Can you work these out from the model? Positions are in its coordinate system, mm. Face numbers are marked on the shaded views. A direction names the side the tool comes from. Coordinates: 2 decimals unless noted, no trailing zeros. Order: outer loops, then holes, each group sorted by start corner. A loop starts at its lowest first (then second) coordinate and runs counter-clockwise, first axis right, second up. Notation, with made-up numbers: (82.25, 80.5) - (102.25, 80.5) arc R19 ccw to (102.25, 113.5) - close; hole circle Ø4 at (16.5, 70.5). An arc over 180 degrees is marked (long way). Use a Markdown table: item, result. Add a question column.
(1) I want a section at B-B (y = 0). List the corners of the cut face in (x, z) for me (3 decimals), and give its area (3 significant figures).
(2) If I drill on L1, parallel to Y at x = 0, z = 15.5; L2, parallel to Z at x = 0, y = 11.5; L3, parallel to Z at x = -14.5, y = -59.5, over which ranges is the centre line in solid material (lowest first)? Write a range as [from, to].
(3) On a 3-axis mill with a long thin cutter (end or side, diameter ignored), from which of +Z, -Z, +X, -X, +Y, -Y can I reach the whole of each face in a straight line? I mean the marked faces 1, 2 and 3. Say none if no direction works.
(4) I want a section at C-C (z = 18). List the corners of the cut face in (x, y) for me.
(5) For pin 1 Ø8 at (y, z) = (32.5, 3) entering from +X; pin 2 Ø16 at (x, y) = (-2.5, -0.5) entering from +Z; pin 3 Ø8 at (y, z) = (-7.5, -5) entering from -X, each with a flat end and sliding along its axis, tell me the tip position at first contact or that it passes through.
(6) I want a section at D-D (z = -14). List the corners of the cut face in (x, y) for me.
Autodesk Inventor part; units mm, degrees
ref_plane "YZ Plane" through (0, 0, 0) normal (1, 0, 0) x (0, 1, 0)
ref_plane "XZ Plane" through (0, 0, 0) normal (0, 1, 0) x (-1, 0, 0)
ref_plane "XY Plane" through (0, 0, 0) normal (0, 0, 1) x (1, 0, 0)
sketch "草图1" plane through (0, 0, 0) normal (0, 0, 1) x (1, 0, 0)
  circle A0 centre (0, 0) radius 65
  dimension "d0" = 130
extrude "拉伸1" add sketch "草图1" along normal blind 12
sketch "草图2" plane through (0, 0, 12) normal (0, 0, 1) x (1, 0, 0)
  circle A0 centre (0, 0) radius 50
  circle A1 centre (0, 50) radius 7.5
  line L0 (0, 0) -> (0, 11.3897)
  dimension "d3" = 100
  dimension "d4" = 15
  dimension "d5" = 11.3897
extrude "拉伸2" add sketch "草图2" along normal blind 15 contours A1 A0 | A0 A1 picked at (0, 47.4583) picked at (0.2152, 52.449)
sketch "草图3" plane through (0, 50, 27) normal (0, 0, 1) x (1, 0, 0)
  circle A0 centre (0, 0) radius 2.5
  circle A1 centre (0, 0) radius 7.5
  point P0 (0, -50)
  dimension "d8" = 5
extrude "拉伸3" cut sketch "草图3" against normal through all contours A0
thread "螺纹1"
sketch "草图4" plane through (0, 0, 0) normal (0, 0, -1) x (-1, 0, 0)
  circle A0 centre (0, 0) radius 10
  dimension "d13" = 20
extrude "拉伸4" add sketch "草图4" along normal blind 59.7
sketch "草图5" plane through (0, 0, 0) normal (0, 0, -1) x (-1, 0, 0)
  circle A0 centre (0, 0) radius 13
  dimension "d16" = 26
extrude "拉伸5" add sketch "草图5" along normal blind 3
chamfer "倒角1" distance 2 angle 45 2 edges at (-65, 0, 0) (-65, 0, 12)
chamfer "倒角2" distance 0.5 angle 45 1 edges at (10, 0, -59.7)
sketch "草图6" plane through (0, 0, 0) normal (0, 1, 0) x (-1, 0, 0)
  line L0 (-9.175, -54.5) -> (-18.451, -54.5)
  line L1 (-18.451, -54.5) -> (-18.451, -55.7)
  line L2 (-18.451, -55.7) -> (-9.175, -55.7)
  line L3 (-9.175, -55.7) -> (-9.175, -54.5)
  line L4 (9.5, -59.7) -> (-9.5, -59.7)
  line L5 (0, -59.7) -> (0, -69.9932)
  point P0 (0, 0)
  dimension "d25" = 10.2932
  dimension "d26" = 4
  dimension "d27" = 1.2
  dimension "d28" = 9.175
  dimension "d29" = 9.276
revolve "旋转1" cut sketch "草图6" angle 360 about axis through (0, 0, -59.7) along (0, 0, -1)
properties part number "刀轴带动盘"
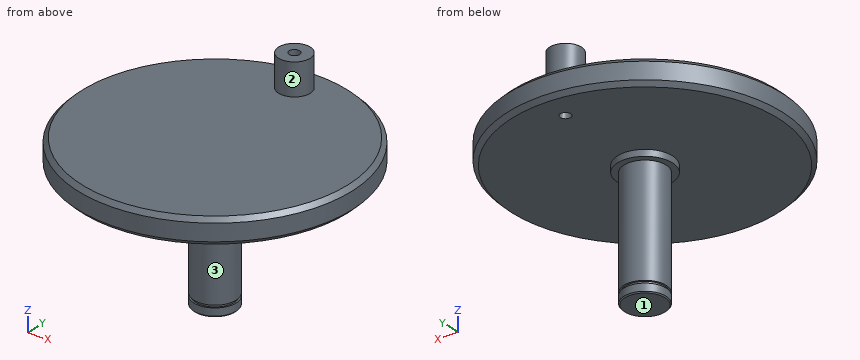
Answers follow:
| question | item | result |
|---|---|---|
| 1 | outline | (-65, 2) - (-63, 0) - (-13, 0) - (-13, -3) - (-10, -3) - (-10, -54.5) - (-9.175, -54.5) - (-9.175, -55.7) - (-10, -55.7) - (-10, -59.2) - (-9.5, -59.7) - (9.5, -59.7) - (10, -59.2) - (10, -55.7) - (9.175, -55.7) - (9.175, -54.5) - (10, -54.5) - (10, -3) - (13, -3) - (13, 0) - (63, 0) - (65, 2) - (65, 10) - (63, 12) - (-63, 12) - (-65, 10) - close |
| 1 | area | 2,760 mm² |
| 2 | L1 | y = [42.5, 47.5], [52.5, 57.5] |
| 2 | L2 | z = [-3, 12] |
| 2 | L3 | z = [0, 12] |
| 3 | face 1 | -Z, +X, -X, +Y, -Y |
| 3 | face 2 | +Z |
| 3 | face 3 | -Z |
| 4 | outline | circle Ø15 at (0, 50); hole circle Ø5 at (0, 50) |
| 5 | pin 1 | stops at x = 58.42 |
| 5 | pin 2 | stops at z = 12 |
| 5 | pin 3 | stops at x = -12.36 |
| 6 | outline | circle Ø20 at (0, 0) |
